Work out the finished part from the listing and answer in its coordinate system (mm). Round coordinates to 2 decimals unless told otherwise and drop trailing zeros. Loops run counter-clockwise (first coordinate to the right, second up) from the corner with the lowest first, then second, coordinate; pieces in that order, holes last. Notation, with made-up numbers: (5.5, -32.75) - (22.5, -32.75) arc R19 cw to (22.5, -20.75) - close; hole circle Ø2 at (83, 78). An arc over 180 degrees is marked (long way). Return JSON: item names as keys, results as strings.
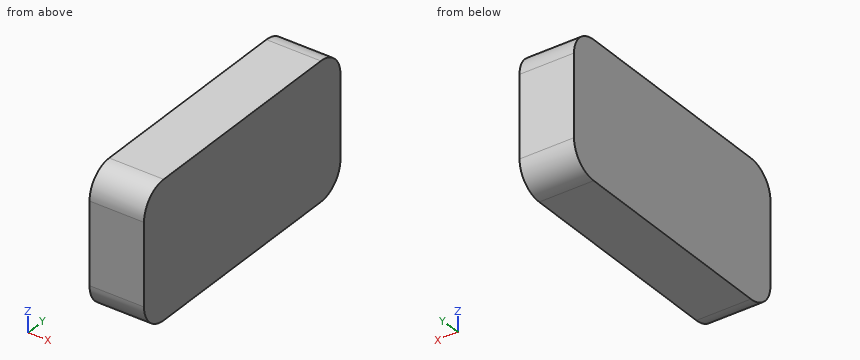
from build123d import *

# Parameters (mm, degrees)
F1_DEPTH = 12.7


with BuildPart() as f1:
    # F0 (on Right) → F1 (new body, symmetric)
    with BuildSketch(Plane.YZ):
        with BuildLine():
            ThreePointArc((63.5, 19.05), (59.780256, 28.030256), (50.8, 31.75))
            Line((50.8, 31.75), (-50.8, 31.75))
            ThreePointArc((-50.8, 31.75), (-59.780256, 28.030256), (-63.5, 19.05))
            Line((-63.5, 19.05), (-63.5, -19.05))
            ThreePointArc((-63.5, -19.05), (-59.780256, -28.030256), (-50.8, -31.75))
            Line((-50.8, -31.75), (50.8, -31.75))
            ThreePointArc((50.8, -31.75), (59.780256, -28.030256), (63.5, -19.05))
            Line((63.5, -19.05), (63.5, 19.05))
        make_face()
    extrude(amount=F1_DEPTH, both=True)


solid = f1.part
1) Section C-C (z = -24.5) is taken. Give the vertices of the cut face in (x, y), and give its area (3 significant figures).
Verdict:
{"outline": "(-12.7, -62.27) - (12.7, -62.27) - (12.7, 62.27) - (-12.7, 62.27) - close", "area": "3,160 mm2"}
2) Flat-ended cylindrical pins translate along their axes: pin 1 (5 mm diameter, centred on x = 6, z = -23.5, fed in from -Y); pin 2 (8 mm diameter, centred on x = -6, z = -19.5, fed in from +Y). Find the tip coordinate at first contact, or state that the pin passes through.
Verdict:
{"pin 1": "stops at y = -63.35", "pin 2": "stops at y = 63.5"}
3) Find the intervals of material crossed by L1, parallel to Z at x = 1.75, y = -52.5; L2, parallel to Y at x = 2.25, z = 24.5; L3, parallel to Y at x = 9.75, z = 20.5, in increasing order.
Verdict:
{"L1": "z = -31.64 to 31.64", "L2": "y = -62.27 to 62.27", "L3": "y = -63.42 to 63.42"}
4) Section A-A (x = -3.5) is taken. Give the vertices of the cut face in (y, z).
Verdict:
{"outline": "(-63.5, -19.05) arc R12.7 ccw to (-50.8, -31.75) - (50.8, -31.75) arc R12.7 ccw to (63.5, -19.05) - (63.5, 19.05) arc R12.7 ccw to (50.8, 31.75) - (-50.8, 31.75) arc R12.7 ccw to (-63.5, 19.05) - close"}
5) Section B-B (z = 27.5) is taken. Give the vertices of the cut face in (x, y), and give its area (3 significant figures).
Verdict:
{"outline": "(-12.7, -60.28) - (12.7, -60.28) - (12.7, 60.28) - (-12.7, 60.28) - close", "area": "3,060 mm2"}
